Here's how the part is built. I have some questions about the finished solid (model axes, mm). Face numbers are marked on the shaded views. A direction names the side the tool comes from. Round coordinates to 2 decimals unless told otherwise and drop trailing zeros. Loops run counter-clockwise (first coordinate to the right, second up) from the corner with the lowest first, then second, coordinate; pieces in that order, holes last. Notation, with made-up numbers: M -15,44 L -4,44 A20 ccw -4,74 Z; hole C 86.25,-24 d3. An arc over 180 degrees is marked long. Write each question's results on one line, items separated by ' | '. Start each with the question number.
```python
from build123d import *

# Parameters (mm, degrees)
SKETCH1_W           = 38.3
SKETCH1_H           = 27
SKETCH1_R           = 4
BOSS_EXTRUDE1_DEPTH = 2
SKETCH2_W           = 4
SKETCH2_H           = 27
BOSS_EXTRUDE2_DEPTH = 64
CUT_EXTRUDE1_REACH  = 6


with BuildPart() as part:
    # Sketch1 → Boss-Extrude1 (new body)
    with BuildSketch(Plane(origin=(0, 0, 0), x_dir=(1, 0, 0), z_dir=(0, 1, 0))):
        Rectangle(SKETCH1_W, SKETCH1_H)
        with Locations((-6.85, 0)):
            Circle(SKETCH1_R, mode=Mode.SUBTRACT)
    extrude(amount=BOSS_EXTRUDE1_DEPTH)

    # Sketch2 → Boss-Extrude2 (add)
    with BuildSketch(Plane(origin=(0, 2, 0), x_dir=(1, 0, 0), z_dir=(0, 1, 0))):
        with Locations((17.15, 0)):
            Rectangle(SKETCH2_W, SKETCH2_H)
    extrude(amount=BOSS_EXTRUDE2_DEPTH)

    # Sketch3 → Cut-Extrude1 (cut, up to next)
    with BuildSketch(Plane.ZY.offset(-15.15), mode=Mode.PRIVATE) as cut_extrude1_sk1:
        with BuildLine():
            Line((-12.5, 14), (-12.5, 54))
            ThreePointArc((-12.5, 54), (-11.125, 55.375), (-9.75, 54))
            Line((-9.75, 54), (-9.75, 14))
            ThreePointArc((-9.75, 14), (-11.125, 12.625), (-12.5, 14))
        make_face()
    cut_extrude1_tool1 = extrude(cut_extrude1_sk1.sketch, amount=-CUT_EXTRUDE1_REACH, mode=Mode.PRIVATE) & part.part
    add(cut_extrude1_tool1.solids().sort_by_distance((15.15, 34, -11.125))[0], mode=Mode.SUBTRACT)
    # Sketch3 → Cut-Extrude1 (cut, up to next)
    with BuildSketch(Plane.ZY.offset(-15.15), mode=Mode.PRIVATE) as cut_extrude1_sk2:
        with BuildLine():
            Line((12.5, 14), (12.5, 54))
            ThreePointArc((12.5, 54), (11.125, 55.375), (9.75, 54))
            Line((9.75, 54), (9.75, 14))
            ThreePointArc((9.75, 14), (11.125, 12.625), (12.5, 14))
        make_face()
    cut_extrude1_tool2 = extrude(cut_extrude1_sk2.sketch, amount=-CUT_EXTRUDE1_REACH, mode=Mode.PRIVATE) & part.part
    add(cut_extrude1_tool2.solids().sort_by_distance((15.15, 34, 11.125))[0], mode=Mode.SUBTRACT)
    # Sketch3 → Cut-Extrude1 (cut, up to next)
    with BuildSketch(Plane.ZY.offset(-15.15), mode=Mode.PRIVATE) as cut_extrude1_sk3:
        with BuildLine():
            Line((-5.125, 14), (-5.125, 56))
            ThreePointArc((-5.125, 56), (0, 61.125), (5.125, 56))
            Line((5.125, 56), (5.125, 14))
            ThreePointArc((5.125, 14), (0, 8.875), (-5.125, 14))
        make_face()
    cut_extrude1_tool3 = extrude(cut_extrude1_sk3.sketch, amount=-CUT_EXTRUDE1_REACH, mode=Mode.PRIVATE) & part.part
    add(cut_extrude1_tool3.solids().sort_by_distance((15.15, 35, 0))[0], mode=Mode.SUBTRACT)


solid = part.part
```
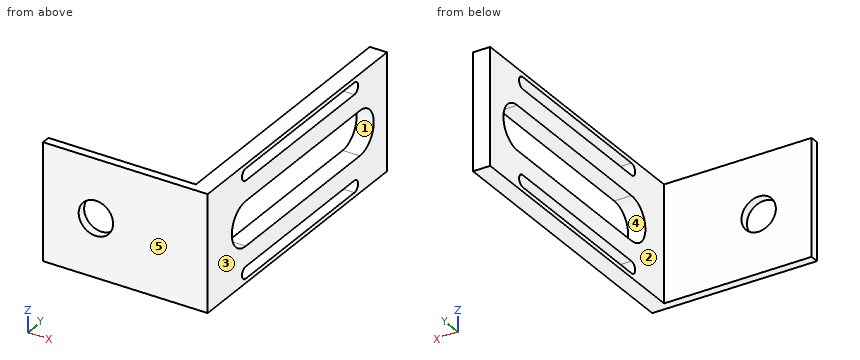
1. I want a section at C-C on y = 30. List the corners of the cut face in (x, z) for me (3 decimals).
2. If we mould it in two halves opening along Z, with no side actions, what happens to the marked faces 4 and 5? For each: released by +Z, released by -Z, zero draft, split by the parting line, or undercut.
3. I want a section at A-A on z = 0. List the corners of the cut face in (x, y) for me (3 decimals), plus the area to 3 significant figures.
4. For pin 1 (13.5 mm diameter, centred on y = 29.5, z = 1, fed in from -X); pin 2 (7 mm diameter, centred on x = -6.85, z = 0, fed in from -Y); pin 3 (12 mm diameter, centred on x = 2, z = -3, fed in from +Y); pin 4 (12 mm diameter, centred on y = 16.5, z = -5.5, fed in from -X), each with a flat end and sliding along its axis, tell me the tip position at first contact or that it passes through.
5. Which directions (+Z, -Z, +X, -X, +Y, -Y) give clear straight access to the entire face, cutting with the end or side of a thin tool? Please do the marked faces 1, 2 and 3.
6. I want a section at B-B on x = -6.85. List the corners of the cut face in (y, z) for me, plus the area to 3 significant figures.
7. I want a section at D-D on z = 11. List the corners of the cut face in (x, y) for me, plus the area to 3 significant figures.
8. I need wall thicknesses on line 1 along Z through (x, y) = (-6.85, 0.6); line 2 along X through (y, z) = (0.95, 0); line 3 along Y through (x, z) = (9, 2). Which ranges of each line are inside material? Lowest first, please.
Outcome:
1) outline: M 15.15,-13.5 L 19.15,-13.5 L 19.15,-12.5 L 15.15,-12.5 Z; M 15.15,-9.75 L 19.15,-9.75 L 19.15,-5.125 L 15.15,-5.125 Z; M 15.15,5.125 L 19.15,5.125 L 19.15,9.75 L 15.15,9.75 Z; M 15.15,12.5 L 19.15,12.5 L 19.15,13.5 L 15.15,13.5 Z
2) face 4: undercut | face 5: zero draft
3) outline: M -19.15,0 L -10.85,0 L -10.85,2 L -19.15,2 Z; M -2.85,0 L 19.15,0 L 19.15,8.875 L 15.15,8.875 L 15.15,2 L -2.85,2 Z; M 15.15,61.125 L 19.15,61.125 L 19.15,66 L 15.15,66 Z | area: 108 mm2
4) pin 1: x = 15.15 | pin 2: through | pin 3: y = 2 | pin 4: x = 15.15
5) face 1: +X, -X | face 2: +Z, -Z, -X, +Y | face 3: +Z, -Z, +X, +Y, -Y
6) outline: M 0,-13.5 L 2,-13.5 L 2,-4 L 0,-4 Z; M 0,4 L 2,4 L 2,13.5 L 0,13.5 Z | area: 38.0 mm2
7) outline: M -19.15,0 L 19.15,0 L 19.15,12.63 L 15.15,12.63 L 15.15,2 L -19.15,2 Z; M 15.15,55.37 L 19.15,55.37 L 19.15,66 L 15.15,66 Z | area: 162 mm2
8) line 1: -13.5 to -4, 4 to 13.5 | line 2: -19.15 to -10.85, -2.85 to 19.15 | line 3: 0 to 2
